```python
from build123d import *

# Parameters (mm, degrees)
BOSS_EXTRUDE1_DEPTH = 3.96875
SKETCH4_W           = 1.7272
SKETCH4_H           = 11.14425
CHAMFER1_SIZE       = 0.381


with BuildPart() as part:
    # Sketch1 → Boss-Extrude1 (new body, symmetric)
    with BuildSketch(Plane.XY):
        with BuildLine():
            Line((-7.84225, 0.762), (-4.701144781, 0.762))
            ThreePointArc((-4.701144781, 0.762), (0, 4.7625), (4.701144781, 0.762))
            Line((4.701144781, 0.762), (11.88184098, 0.762))
            ThreePointArc((11.88184098, 0.762), (-11.90625, 0), (11.88184098, -0.762))
            Line((11.88184098, -0.762), (4.701144781, -0.762))
            ThreePointArc((4.701144781, -0.762), (0, -4.7625), (-4.701144781, -0.762))
            Line((-4.701144781, -0.762), (-7.84225, -0.762))
            Line((-7.84225, -0.762), (-7.84225, 0.762))
        make_face()
    extrude(amount=BOSS_EXTRUDE1_DEPTH, both=True)

    # Sketch4 → #8-32 Tapped Hole1 (revolve, cut)
    with BuildSketch(Plane(origin=(8.29149288, -0.762, 0), x_dir=(0, 0, 1), z_dir=(1, 0, 0))):
        with Locations((0.8636, 5.572125)):
            Rectangle(SKETCH4_W, SKETCH4_H)
    revolve(axis=Axis((8.29149288, 5.588, 0), (0, -1, 0)), mode=Mode.SUBTRACT)

    # Chamfer1
    chamfer1_edges = [part.edges().sort_by_distance(p)[0] for p in [
        (0, -4.7625, -3.96875),
        (0, 4.7625, 3.96875),
        (-11.90625, 0, 3.96875),
        (0, -4.7625, 3.96875),
        (-11.90625, 0, -3.96875),
        (0, 4.7625, -3.96875),
    ]]
    chamfer(chamfer1_edges, length=CHAMFER1_SIZE)

    # Sketch10 → Cut-Revolve1 (revolve, cut)
    with BuildSketch(Plane.XY):
        Polygon((8.29149288, 0.762), (10.50129288, 0.762), (10.50129288, 3.048), (11.97449288, 3.048), (11.97449288, 11.90625), (8.29149288, 11.90625), align=None)
    revolve(axis=Axis((8.29149288, -0.762, 0), (0, -1, 0)), mode=Mode.SUBTRACT)


solid = part.part
```
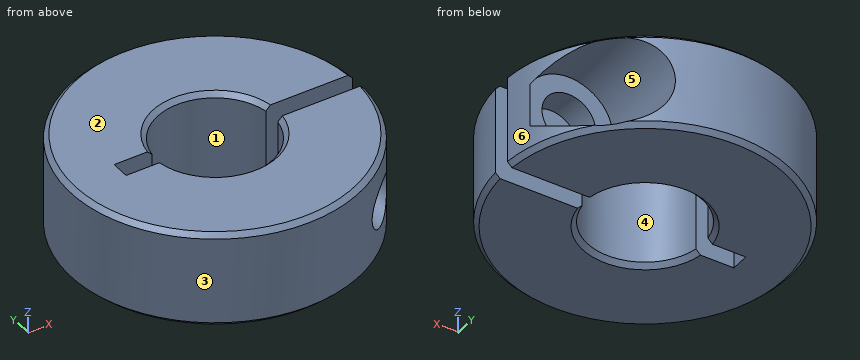
Source: CAD feature listing. Evaluate the final solid. Frame: model axes, mm. Face numbers are marked on the shaded views. A direction names the side the tool comes from. Round coordinates to 2 decimals unless told otherwise and drop trailing zeros. Write each loop counter-clockwise with the first axis right and the second up, starting at its lowest first coordinate (ties: lowest second). Pieces come first, ordered by that corner, then holes. Notation, with made-up numbers: M -37.75,69 L 11.25,69 A33 ccw 11.25,98 Z; hole C 43,25.25 d1. An arc over 180 degrees is marked long. Answer as a JSON object with one key per item and string values. Group by question number.
(1) Reachability of the marked faces 4, 5 and 6 from +Z, -Z, +X, -X, +Y, -Y: full face, straight path, thin tool, end or side. Return the list, or none.
(2) Section query D-D on z = -2.5. Output: boundary loops of the cut face in (x, y) (1 decimal), then the cut area to 3 significant figures.
(3) Ray query, line 1 (X direction, y = -2.25, z = 3); line 2 (Z direction, x = 10, y = 3); line 3 (Y direction, x = -4.25, z = 3.75). Return the intervals inside material, ascending. Write a range as [from, to].
(4) Mould query, pull axis Y, two halves, no side actions, for the marked faces 1, 2 and 3. Classes: +Y half, -Y half, draft (parallel to the pull), parting line (faces both ways), or undercut.
(5) Section query B-B on z = 0. Output: boundary loops of the cut face in (x, y) (1 decimal), then the cut area to 3 significant figures.
(6) First-contact query: pin 1 (1.5 mm diameter, centred on y = -7, z = 1, fed in from -X); pin 2 (1.5 mm diameter, centred on y = -4, z = -1, fed in from +X); pin 3 (2 mm diameter, centred on x = 6.5, z = 2, fed in from -Y); pin 4 (3 mm diameter, centred on x = 8.29, z = 0, fed in from +Y). Flat tips, straight axial feed; report the tip coordinate or a pass-through.
(7) Section query A-A on x = 0. Output: boundary loops of the cut face in (y, z).
(8) Section query C-C on y = 0. Output: boundary loops of the cut face in (x, z), then the cut area to 3 significant figures.
Computed values:
{
 "1": {"face 4": "+Z, -Z", "face 5": "+Y", "face 6": "+Z, -Z, +X, +Y"},
 "2": {"outline": "M -7.8,-0.8 L -7.8,0.8 L -4.7,0.8 A4.8 cw 4.7,0.8 L 11.9,0.8 A11.9 ccw 11,4.6 L 11,3 L 5.6,3 L 5.6,10.5 A11.9 ccw long 11.9,-0.8 L 4.7,-0.8 A4.8 cw -4.7,-0.8 Z", "area": "330 mm^2"},
 "3": {"line 1": "[-11.69, -4.2], [4.2, 11.69]", "line 2": "[-3.97, -1.4], [1.4, 3.97]", "line 3": "[-10.95, -2.49], [2.49, 10.95]"},
 "4": {"face 1": "undercut", "face 2": "draft", "face 3": "parting line"},
 "5": {"outline": "M -7.8,-0.8 L -7.8,0.8 L -4.7,0.8 A4.8 cw 4.7,0.8 L 6.1,0.8 L 6.1,3 L 4.6,3 L 4.6,11 A11.9 ccw long 6.6,-9.9 L 6.6,-0.8 L 4.7,-0.8 A4.8 cw -4.7,-0.8 Z; M 10,-6.4 A11.9 ccw 11.9,-0.8 L 10,-0.8 Z; M 10.5,0.8 L 11.9,0.8 A11.9 ccw 11.5,3 L 10.5,3 Z", "area": "286 mm^2"},
 "6": {"pin 1": "x = -10.13", "pin 2": "x = 11.45", "pin 3": "y = -10.56", "pin 4": "through"},
 "7": {"outline": "M -11.91,-3.59 L -11.53,-3.97 L -5.14,-3.97 L -4.76,-3.59 L -4.76,3.59 L -5.14,3.97 L -11.53,3.97 L -11.91,3.59 Z; M 4.76,-3.59 L 5.14,-3.97 L 11.53,-3.97 L 11.91,-3.59 L 11.91,3.59 L 11.53,3.97 L 5.14,3.97 L 4.76,3.59 Z"},
 "8": {"outline": "M -11.91,-3.59 L -11.53,-3.97 L -7.84,-3.97 L -7.84,3.97 L -11.53,3.97 L -11.91,3.59 Z", "area": "32.1 mm^2"}
}
